from build123d import *

# Parameters (mm, degrees)
SKETCH021_W     = 117
SKETCH021_H     = 85
PAD012_DEPTH    = 17.8
SKETCH025_W     = 111.4
SKETCH025_H     = 79.4
POCKET003_DEPTH = 15.8
SKETCH026_W     = 4
SKETCH026_H     = 79.4
PAD014_DEPTH    = 6.5
SKETCH027_W     = 4
SKETCH027_H     = 8
POCKET004_DEPTH = 2
SKETCH028_W     = 13
SKETCH028_H     = 6
SKETCH028_W_2   = 5.8
SKETCH028_H_2   = 4
SKETCH028_W_3   = 4
SKETCH028_H_3   = 1.6
POCKET005_DEPTH = 2.8
SKETCH029_W     = 0.6
SKETCH029_H     = 28.3
POCKET006_DEPTH = 7.8
SKETCH030_W     = 13
SKETCH030_H     = 2
POCKET007_DEPTH = 2.8
SKETCH032_R     = 1.2
POCKET009_DEPTH = 2.8
SKETCH037_W     = 10
SKETCH037_H     = 8
POCKET012_DEPTH = 5
POCKET015_DEPTH = 85.001
SKETCH056_W     = 1
SKETCH056_H     = 47.4
SKETCH056_H_2   = 16
PAD026_DEPTH    = 1.5
SKETCH057_W     = 0.6
SKETCH057_H     = 0.3
POCKET019_DEPTH = 7.8
POCKET020_DEPTH = 2.8
SKETCH059_W     = 13
SKETCH059_H     = 5
POCKET021_DEPTH = 2.8


with BuildPart() as part:
    # Sketch021 → Pad012 (new body)
    with BuildSketch(Plane.XY):
        with Locations((0.5, -8)):
            Rectangle(SKETCH021_W, SKETCH021_H)
    extrude(amount=PAD012_DEPTH)

    # Sketch025 (on Face6 of Pad012) → Pocket003 (cut)
    with BuildSketch(Plane.XY.offset(17.8)):
        with Locations((0.5, -8)):
            Rectangle(SKETCH025_W, SKETCH025_H)
    extrude(amount=-POCKET003_DEPTH, mode=Mode.SUBTRACT)

    # Sketch026 (on Face11 of Pocket003) → Pad014 (join)
    with BuildSketch(Plane.XY.offset(2)):
        with Locations((-53.2, -8)):
            Rectangle(SKETCH026_W, SKETCH026_H)
        with Locations((54.2, -8)):
            Rectangle(SKETCH026_W, SKETCH026_H)
    extrude(amount=PAD014_DEPTH)

    # Sketch027 (on Face15 of Pad014) → Pocket004 (cut)
    with BuildSketch(Plane.XY.offset(8.5)):
        with Locations((-53.2, 27.7)):
            Rectangle(SKETCH027_W, SKETCH027_H)
        with Locations((54.2, 27.7)):
            Rectangle(SKETCH027_W, SKETCH027_H)
        with Locations((-53.2, -27.7)):
            Rectangle(SKETCH027_W, SKETCH027_H)
        with Locations((54.2, -27.7)):
            Rectangle(SKETCH027_W, SKETCH027_H)
    extrude(amount=-POCKET004_DEPTH, mode=Mode.SUBTRACT)

    # Sketch028 (on Face3 of Pocket004) → Pocket005 (cut)
    with BuildSketch(Plane.YZ.offset(59)):
        with Locations((-13, 14.8)):
            Rectangle(SKETCH028_W, SKETCH028_H)
        with Locations((-1.3, 15.8)):
            Rectangle(SKETCH028_W_2, SKETCH028_H_2)
        with Locations((6.5, 15.8)):
            Rectangle(SKETCH028_W_3, SKETCH028_H_2)
        with Locations((18.5, 15.8)):
            Rectangle(SKETCH028_W_3, SKETCH028_H_2)
        with Locations((12.5, 15.8)):
            Rectangle(SKETCH028_W_3, SKETCH028_H_3)
    extrude(amount=-POCKET005_DEPTH, mode=Mode.SUBTRACT)

    # Sketch029 (on Face18 of Pocket005) → Pocket006 (cut)
    with BuildSketch(Plane.XY.offset(17.8)):
        with Locations((56.5, 7.95)):
            Rectangle(SKETCH029_W, SKETCH029_H)
    extrude(amount=-POCKET006_DEPTH, mode=Mode.SUBTRACT)

    # Sketch030 (on Face1 of Pocket006) → Pocket007 (cut)
    with BuildSketch(Plane(origin=(0, 34.5, 0), x_dir=(-1, 0, 0), z_dir=(0, 1, 0))):
        with Locations((-37.9, 15.6)):
            Rectangle(SKETCH030_W, SKETCH030_H)
    extrude(amount=-POCKET007_DEPTH, mode=Mode.SUBTRACT)

    # Sketch032 (on Face13 of Pocket007) → Pocket009 (cut)
    with BuildSketch(Plane(origin=(0, -47.7, 0), x_dir=(-1, 0, 0), z_dir=(0, 1, 0))):
        with Locations((-48.2, 4)):
            Circle(SKETCH032_R)
        with Locations((-43.2, 4)):
            Circle(SKETCH032_R)
    extrude(amount=-POCKET009_DEPTH, mode=Mode.SUBTRACT)

    # Sketch037 (on Face4 of Pocket009) → Pocket012 (cut)
    with BuildSketch(Plane.XY.offset(17.8)):
        with Locations((-53, 30.5)):
            Rectangle(SKETCH037_W, SKETCH037_H)
        with Locations((54, 30.5)):
            Rectangle(SKETCH037_W, SKETCH037_H)
        with Locations((-53, -46.5)):
            Rectangle(SKETCH037_W, SKETCH037_H)
        with Locations((54, -46.5)):
            Rectangle(SKETCH037_W, SKETCH037_H)
    extrude(amount=-POCKET012_DEPTH, mode=Mode.SUBTRACT)

    # Sketch043 (on Face14 of Pocket012) → Pocket015 (cut, through all)
    with BuildSketch(Plane.XZ.offset(50.5)):
        Polygon((-48, 12.8), (-46.6, 12.8), (-46.6, 14.4), (-48, 16), align=None)
        Polygon((49, 12.8), (47.6, 12.8), (47.6, 14.4), (49, 16), align=None)
    extrude(amount=-POCKET015_DEPTH, mode=Mode.SUBTRACT)

    # Sketch056 (on Face70 of Pocket015) → Pad026 (join)
    with BuildSketch(Plane.XY.offset(8.5)):
        with Locations((55.7, 0)):
            Rectangle(SKETCH056_W, SKETCH056_H)
        with Locations((55.7, -39.7)):
            Rectangle(SKETCH056_W, SKETCH056_H_2)
    extrude(amount=PAD026_DEPTH)

    # Sketch057 (on Face27 of Pad026) → Pocket019 (cut)
    with BuildSketch(Plane.XY.offset(17.8)):
        with Locations((56.5, -6.35)):
            Rectangle(SKETCH057_W, SKETCH057_H)
    extrude(amount=-POCKET019_DEPTH, mode=Mode.SUBTRACT)

    # Sketch058 (on Face15 of Pocket019) → Pocket020 (cut)
    with BuildSketch(Plane(origin=(-58, 0, 0), x_dir=(0, -1, 0), z_dir=(-1, 0, 0))):
        with BuildLine():
            ThreePointArc((-8, 13.2), (-8.6, 12.6), (-8, 12))
            Line((-8, 12), (-2, 12))
            ThreePointArc((-2, 12), (-1.4, 12.6), (-2, 13.2))
            Line((-8, 13.2), (-2, 13.2))
        make_face()
        with BuildLine():
            ThreePointArc((2, 13.2), (1.4, 12.6), (2, 12))
            Line((2, 12), (8, 12))
            ThreePointArc((8, 12), (8.6, 12.6), (8, 13.2))
            Line((2, 13.2), (8, 13.2))
        make_face()
    extrude(amount=-POCKET020_DEPTH, mode=Mode.SUBTRACT)

    # Sketch059 (on Face20 of Pocket020) → Pocket021 (cut)
    with BuildSketch(Plane.XZ.offset(50.5)):
        with Locations((-18.9, 15.3)):
            Rectangle(SKETCH059_W, SKETCH059_H)
    extrude(amount=-POCKET021_DEPTH, mode=Mode.SUBTRACT)


solid = part.part
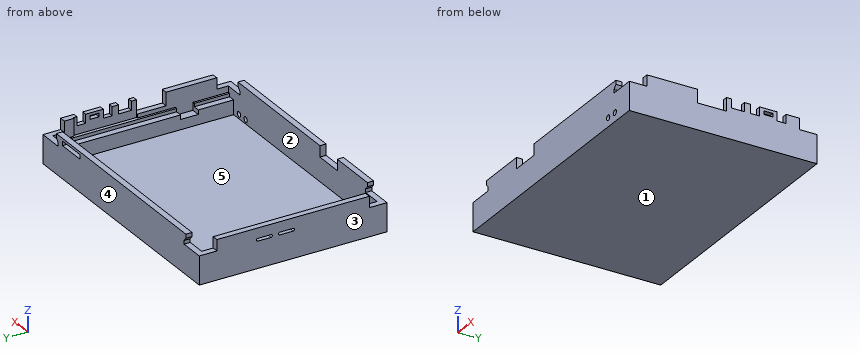
Model file for the job. Use its own axes, mm. Face numbers are marked on the shaded views. A direction names the side the tool comes from. Coordinates: 2 decimals unless noted, no trailing zeros. Write each loop counter-clockwise with the first axis right and the second up, starting at its lowest first coordinate (ties: lowest second). Pieces come first, ordered by that corner, then holes. Notation, with made-up numbers: (2.25, 39.5) - (45.25, 39.5) arc R9 cw to (45.25, 43.5) - close; hole circle Ø1 at (64, -8.5). An arc over 180 degrees is marked (long way). Write each question's results on one line, items separated by ' | '. Start each with the question number.
1) Flat gauge pins, fed straight in: P1, Ø2, axis at x = -57, z = 15.5, coming from the -Y side; P2, Ø1.4, axis at x = -57, z = 14.5, coming from the +Y side; P3, Ø3, axis at x = 57, y = -15.5, coming from the +Z side; P4, Ø2, axis at x = 38.5, y = 33, coming from the -Z side. Where does each tip first touch, or does it go through?
2) Mould opens along X. For the marked faces 1, 2 and 3 say: pulls with the +X half, pulls with the -X half, needs draft (parallel to the pull), parting line crosses it, or undercut.
3) Cut at C-C (x = -38.5). Write the cut outline in (y, z).
4) Cut at B-B (y = 13). Write the cut outline in (x, z), then the cut area to 3 significant figures.
5) Probe line 1 along X through (y, z) = (-28, 15); line 2 along X through (y, z) = (-4.5, 4); line 3 along Z through (x, y) = (43.2, -49.1). List the from-to ranges inside material, lowest first. Write a range as from..to.
6) Cut at D-D (y = -29.5). Write the cut outline in (x, z), then the cut area to 3 significant figures.
7) Cut at A-A (z = 4). Write the cut outline in (x, y), then the cut area to 3 significant figures.
8) 3-axis set-ups, long thin cutter, end or side, ignore diameter. For the marked faces 4 and 5: which of +Z, -Z, +X, -X, +Y, -Y reach the whole face in a straight line?
Returned:
1) P1: y = -42.5 | P2: y = 26.5 | P3: z = 11.8 | P4: z = 0
2) face 1: needs draft | face 2: undercut | face 3: pulls with the -X half
3) outline: (-50.5, 0) - (34.5, 0) - (34.5, 17.8) - (31.7, 17.8) - (31.7, 2) - (-47.7, 2) - (-47.7, 17.8) - (-50.5, 17.8) - close
4) outline: (-58, 0) - (59, 0) - (59, 15) - (56.8, 15) - (56.8, 10) - (55.2, 10) - (55.2, 8.5) - (52.2, 8.5) - (52.2, 2) - (-51.2, 2) - (-51.2, 8.5) - (-55.2, 8.5) - (-55.2, 17.8) - (-58, 17.8) - close; (56.8, 16.6) - (59, 16.6) - (59, 17.8) - (56.8, 17.8) - close | area: 368 mm^2
5) line 1: -58..-55.2, 56.2..59 | line 2: -58..-51.2, 52.2..59 | line 3: 0..2.8, 5.2..17.8
6) outline: (-58, 0) - (59, 0) - (59, 17.8) - (56.2, 17.8) - (56.2, 6.5) - (52.2, 6.5) - (52.2, 2) - (-51.2, 2) - (-51.2, 6.5) - (-55.2, 6.5) - (-55.2, 17.8) - (-58, 17.8) - close | area: 358 mm^2
7) outline: (-58, -50.5) - (42, -50.5) - (42, -47.7) - (-51.2, -47.7) - (-51.2, 31.7) - (52.2, 31.7) - (52.2, -47.7) - (49.4, -47.7) - (49.4, -50.5) - (59, -50.5) - (59, 34.5) - (-58, 34.5) - close; (44.4, -50.5) - (47, -50.5) - (47, -47.7) - (44.4, -47.7) - close | area: 1,720 mm^2
8) face 4: +Z, -Z, +X, -X, +Y | face 5: +Z
